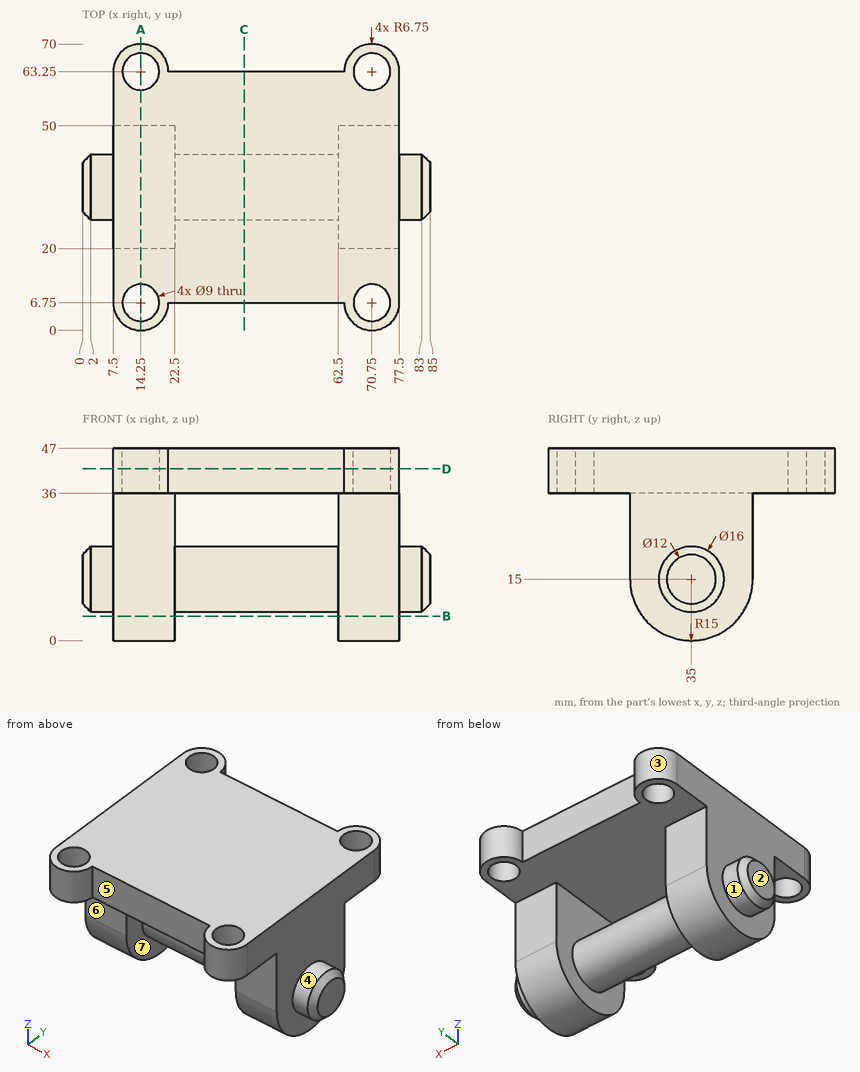
Input: dimensioned drawing with shaded views. Units: mm. Origin: part minimum x, y, z. A direction names the side the tool comes from. Give positions to 0.01 mm unless a question says otherwise; leave off trailing zeros. Write each loop counter-clockwise with the first axis right and the second up, starting at its lowest first coordinate (ties: lowest second). Pieces come first, ordered by that corner, then holes. Notation, with made-up numbers: (31.25, 76) - (78.25, 76) arc R26 cw to (78.25, 112) - close; hole circle Ø2 at (-36.5, 89). An arc over 180 degrees is marked (long way). Write item = value, one per line. Start each with the question number.
1) Reachability of the marked faces 4, 5, 6 and 7 from +Z, -Z, +X, -X, +Y, -Y: full face, straight path, thin tool, end or side. Return the list, or none.
2) Draft query along X for the marked faces 1, 2 and 3. Return one class per face: pulls with the +X half, pulls with the -X half, needs draft (parallel to the pull), parting line crosses it, or undercut.
3) Cut plane C-C (x = 39.5). Return loops of the section in (y, z).
4) Cut plane A-A (x = 14.25). Return loops of the section in (y, z), and give its area (3 significant figures).
5) Cut plane D-D (z = 42). Return loops of the section in (x, y), and give its area (3 significant figures).
6) Cut plane B-B (z = 6). Return loops of the section in (x, y), and give its area (3 significant figures).
7) Pin query (flat end, axial travel): pin 1 (8 mm diameter, centred on y = 23.5, z = 10, fed in from +X); pin 2 (4 mm diameter, centred on x = 67.5, z = 33, fed in from +Y); pin 3 (6 mm diameter, centred on x = 13.5, y = 58.5, fed in from -Z); pin 4 (5.5 mm diameter, centred on x = 14.25, y = 6.75, fed in from +Z). Return the tip coordinate at first contact, or that it passes through.
8) Material intervals for L1, parallel to Y at x = 70.75, z = 42; L2, parallel to X at y = 46.5, z = 21.5; L3, parallel to Z at x = 45, y = 59.5, sorted ascending. Write a range as [from, to].
Answers follow:
q1.face_4 = +X
q1.face_5 = +Z, -Z, -Y
q1.face_6 = -Z, +X, -X, -Y
q1.face_7 = none
q2.face_1 = needs draft
q2.face_2 = pulls with the -X half
q2.face_3 = undercut
q3.outline = (6.75, 36) - (63.25, 36) - (63.25, 47) - (6.75, 47) - close; circle Ø16 at (35, 15)
q4.outline = (0, 36) - (2.25, 36) - (2.25, 47) - (0, 47) - close; (11.25, 36) - (20, 36) - (20, 15) arc R15 ccw to (50, 15) - (50, 36) - (58.75, 36) - (58.75, 47) - (11.25, 47) - close; (67.75, 36) - (70, 36) - (70, 47) - (67.75, 47) - close
q4.area = 1,560 mm^2
q5.outline = (7.5, 6.75) arc R6.75 ccw to (21, 6.75) - (64, 6.75) arc R6.75 ccw to (77.5, 6.75) - (77.5, 63.25) arc R6.75 ccw to (64, 63.25) - (21, 63.25) arc R6.75 ccw to (7.5, 63.25) - close; hole circle Ø9 at (14.25, 6.75); hole circle Ø9 at (14.25, 63.25); hole circle Ø9 at (70.75, 6.75); hole circle Ø9 at (70.75, 63.25)
q5.area = 3,990 mm^2
q6.outline = (7.5, 23) - (22.5, 23) - (22.5, 47) - (7.5, 47) - close; (62.5, 23) - (77.5, 23) - (77.5, 47) - (62.5, 47) - close
q6.area = 720 mm^2
q7.pin_1 = 77.5
q7.pin_2 = 50
q7.pin_3 = 36
q7.pin_4 = through
q8.L1 = [0, 2.25], [11.25, 58.75], [67.75, 70]
q8.L2 = [7.5, 22.5], [62.5, 77.5]
q8.L3 = [36, 47]
